from build123d import *

# Parameters (mm, degrees)
SKETCH1_W               = 1220
SKETCH1_H               = 22.5
BOSS_EXTRUDE1_DEPTH     = 2.5
SKETCH2_W               = 1220
SKETCH2_H               = 2.5
BOSS_EXTRUDE2_DEPTH     = 20
CUT_EXTRUDE1_DEPTH      = 611.742376129
CUT_EXTRUDE1_DEPTH_BACK = 25
FILLET2_R               = 1


with BuildPart() as part:
    # Sketch1 → Boss-Extrude1 (new body)
    with BuildSketch(Plane(origin=(0, 0, 0), x_dir=(1, 0, 0), z_dir=(0, 1, 0))):
        Rectangle(SKETCH1_W, SKETCH1_H)
    extrude(amount=BOSS_EXTRUDE1_DEPTH)

    # Sketch2 → Boss-Extrude2 (add)
    with BuildSketch(Plane(origin=(0, 2.5, 0), x_dir=(1, 0, 0), z_dir=(0, 1, 0))):
        with Locations((0, 10)):
            Rectangle(SKETCH2_W, SKETCH2_H)
    extrude(amount=BOSS_EXTRUDE2_DEPTH)

    # Sketch3 → Cut-Extrude1 (cut, two sides: drawn at the far end of the back side and taken through both)
    with BuildSketch(Plane.XY.offset(-8.75).offset(-CUT_EXTRUDE1_DEPTH_BACK)):
        Polygon((-610, 22.5), (-610, -7.5), (-580, 22.5), align=None)
        Polygon((610, 22.5), (610, -7.5), (580, 22.5), align=None)
    extrude(amount=CUT_EXTRUDE1_DEPTH + CUT_EXTRUDE1_DEPTH_BACK, mode=Mode.SUBTRACT)

    # Fillet2
    fillet2_edges = [part.edges().sort_by_distance(p)[0] for p in [
        (0, 22.5, -8.75),
        (0, 2.5, -8.75),
        (0, 0, 11.25),
        (0, 2.5, 11.25),
        (0, 22.5, -11.25),
        (0, 0, -11.25),
    ]]
    fillet(fillet2_edges, radius=FILLET2_R)


solid = part.part
The listing builds one solid part. Answer for the finished solid, in the listing's coordinates (mm). Coordinates: 2 decimals unless noted, no trailing zeros. Write each loop counter-clockwise with the first axis right and the second up, starting at its lowest first coordinate (ties: lowest second). Pieces come first, ordered by that corner, then holes. Notation, with made-up numbers: (79.5, 47) - (99.5, 47) arc R18 ccw to (99.5, 64) - close; hole circle Ø10 at (45, 43.25). An arc over 180 degrees is marked (long way). Return JSON: item names as keys, results as strings.
1. The part is cut by section A-A on x = -497.5. Determine the outline of the cut face in (y, z).
Final values:
{"outline": "(0, -10.25) arc R1 ccw to (1, -11.25) - (21.5, -11.25) arc R1 ccw to (22.5, -10.25) - (22.5, -9.75) arc R1 ccw to (21.5, -8.75) - (3.5, -8.75) arc R1 cw to (2.5, -7.75) - (2.5, 10.25) arc R1 ccw to (1.5, 11.25) - (1, 11.25) arc R1 ccw to (0, 10.25) - close"}
2. The part is cut by section C-C on z = 0. Determine the outline of the cut face in (x, y), then the cut area to 3 significant figures.
Final values:
{"outline": "(-602.5, 0) - (602.5, 0) - (600, 2.5) - (-600, 2.5) - close", "area": "3,010 mm^2"}
3. The part is cut by section B-B on y = 16. Determine the outline of the cut face in (x, z), then the cut area to 3 significant figures.
Final values:
{"outline": "(-586.5, -11.25) - (586.5, -11.25) - (586.5, -8.75) - (-586.5, -8.75) - close", "area": "2,930 mm^2"}
4. Consider line 1 along Z through (x, y) = (-426.5, 13); line 2 along Y through (x, z) = (23.5, -6); line 3 along X through (y, z) = (2.5, -9). Determine where each line is inside the solid, lowest interval first.
Final values:
{"line 1": "-11.25 to -8.75", "line 2": "0 to 2.5", "line 3": "-600 to 600"}
5. Each of these flat-tipped pins is pushed along its axis until it touches: pin 1 Ø5.5 at (x, z) = (-125, 2) entering from +Y; pin 2 Ø5.5 at (x, y) = (7.5, 10.5) entering from +Z. Where does it stop, or does it pass through?
Final values:
{"pin 1": "y = 2.5", "pin 2": "z = -8.75"}
